from build123d import *

# Parameters (mm, degrees)
SKETCH1_R           = 4.45
SKETCH2_R           = 3.7
SKETCH3_R           = 2.4
SKETCH3_R_2         = 1.7
BOSS_EXTRUDE1_DEPTH = 1.7
SKETCH4_R           = 3.450229513
CUT_EXTRUDE1_DEPTH  = 2.4
SKETCH5_R           = 2.450229513
CUT_EXTRUDE2_DEPTH  = 3.1


with BuildPart() as part:
    # Sketch1 → Loft1 section 0
    with BuildSketch(Plane(origin=(0, 0, 0), x_dir=(1, 0, 0), z_dir=(0, 1, 0))):
        Circle(SKETCH1_R)
    # Sketch2 → Loft1 section 1
    with BuildSketch(Plane(origin=(0, 6.3, 0), x_dir=(1, 0, 0), z_dir=(0, 1, 0))):
        Circle(SKETCH2_R)
    loft()

    # Sketch3 → Boss-Extrude1 (add)
    with BuildSketch(Plane(origin=(0, 6.3, 0), x_dir=(1, 0, 0), z_dir=(0, 1, 0))):
        with Locations(Location((0, 0, 0), (0, 0, 270))):
            Circle(SKETCH3_R)
        with Locations(Location((0, 0, 0), (0, 0, 270))):
            Circle(SKETCH3_R_2, mode=Mode.SUBTRACT)
    extrude(amount=BOSS_EXTRUDE1_DEPTH)

    # Sketch4 → Cut-Extrude1 (cut)
    with BuildSketch(Plane.XZ):
        with Locations(Location((0, 0, 0), (0, 0, 270))):
            Circle(SKETCH4_R)
    extrude(amount=-CUT_EXTRUDE1_DEPTH, mode=Mode.SUBTRACT)

    # Sketch5 → Cut-Extrude2 (cut)
    with BuildSketch(Plane.XZ.offset(-2.4)):
        with Locations(Location((0, 0, 0), (0, 0, 270))):
            Circle(SKETCH5_R)
    extrude(amount=-CUT_EXTRUDE2_DEPTH, mode=Mode.SUBTRACT)


solid = part.part
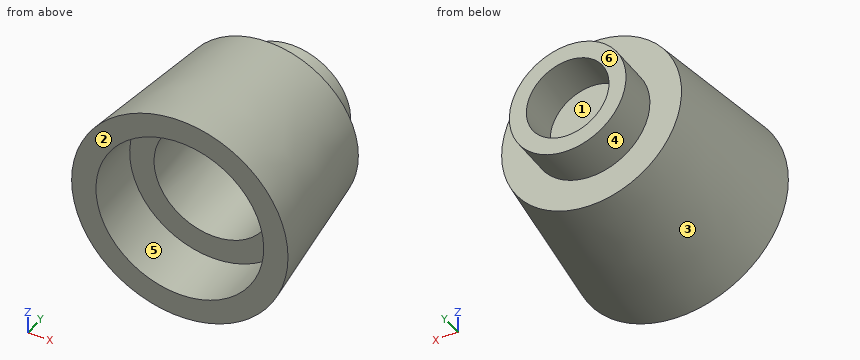
Build history of the part. All positions in model axes, mm. Face numbers are marked on the shaded views. A direction names the side the tool comes from. Coordinates: 2 decimals unless noted, no trailing zeros. Write each loop counter-clockwise with the first axis right and the second up, starting at its lowest first coordinate (ties: lowest second). Pieces come first, ordered by that corner, then holes. Notation, with made-up numbers: (1, 55) -> (32, 55) arc R20 cw to (32, 93) -> close; hole circle Ø2 at (-15.5, -13.5). An arc over 180 degrees is marked (long way). Use CSV: the item, a comma, the result in double quotes. Start each with the question number.
Q1. Cut at C-C, the plane y = 1.5. List the corners of the cut face in (x, z).
Q2. Flat gauge pins, fed straight in: pin 1 Ø1 at (x, y) = (0, 6) entering from +Z; pin 2 Ø1.5 at (x, y) = (-0.5, 1.5) entering from -Z; pin 3 Ø4 at (x, z) = (0, -1) entering from -Y. Where does each tip first touch, or does it go through?
Q3. Drill centre lines: probe 1 along X at (y, z) = (6.9, 0); probe 2 along Y at (x, z) = (3, -0.25); probe 3 along X at (y, z) = (3.4, 0). Where is each one in solid material? Low to high.
Q4. 3-axis set-ups, long thin cutter, end or side, ignore diameter. For the marked faces 4, 5 and 6: which of +Z, -Z, +X, -X, +Y, -Y reach the whole face in a straight line?
Q5. Pull direction Z, two halves, no side cores. Call the marked faces 1, 2 and 3: released by +Z, released by -Z, zero draft, split by the parting line, or undercut.
Q6. Cut at B-B, the plane y = 3.75. List the corners of the cut face in (x, z), then the cut area to 3 significant figures.
Q7. Cut at A-A, the plane x = 0. List the corners of the cut face in (y, z).
Checked values:
1,outline,"circle Ø8.54 at (0, 0); hole circle Ø6.9 at (0, 0)"
2,pin 1,"stops at z = 3.8"
2,pin 2,"stops at z = -4.35"
2,pin 3,"stops at y = 2.4"
3,probe 1,"x = -2.4 to -1.7, 1.7 to 2.4"
3,probe 2,"y = 2.4 to 6.3"
3,probe 3,"x = -4.05 to -2.45, 2.45 to 4.05"
4,face 4,"+Y"
4,face 5,"-Y"
4,face 6,"+Z, -Z, +X, -X, +Y"
5,face 1,"undercut"
5,face 2,"zero draft"
5,face 3,"split by the parting line"
6,outline,"circle Ø8.01 at (0, 0); hole circle Ø4.9 at (0, 0)"
6,area,"31.5 mm²"
7,outline,"(0, -4.45) -> (6.3, -3.7) -> (6.3, -2.4) -> (8, -2.4) -> (8, -1.7) -> (6.3, -1.7) -> (6.3, 1.7) -> (8, 1.7) -> (8, 2.4) -> (6.3, 2.4) -> (6.3, 3.7) -> (0, 4.45) -> (0, 3.45) -> (2.4, 3.45) -> (2.4, 2.45) -> (5.5, 2.45) -> (5.5, -2.45) -> (2.4, -2.45) -> (2.4, -3.45) -> (0, -3.45) -> close"
